Input: part model. Units: mm. Frame: model coordinates. Face numbers are marked on the shaded views. A direction names the side the tool comes from. Give positions to 0.01 mm unless a question says otherwise; leave off trailing zeros. Loops run counter-clockwise (first coordinate to the right, second up) from the corner with the lowest first, then second, coordinate; pieces in that order, holes last. Notation, with made-up numbers: (63, -6.5) -> (99, -6.5) arc R16 cw to (99, 13.5) -> close; hole circle Ø1 at (-28.75, -11). An arc over 180 degrees is marked (long way). Use CSV: the item, a comma, the result in double quotes.
```python
from build123d import *

# Parameters (mm, degrees)
SKETCH_1_R          = 10
SKETCH_1_R_2        = 1.5
EXTRUDE_1_DEPTH     = 4.2
SKETCH_2_R          = 10
SKETCH_2_R_2        = 4.5
SKETCH_2_R_3        = 1.5
SKETCH_2_R_4        = 2.5
CUT_EXTRUDE_1_DEPTH = 2.2


with BuildPart() as part:
    # 草图1 → 凸台-拉伸1 (new body)
    with BuildSketch(Plane(origin=(0, 0, 0), x_dir=(1, 0, 0), z_dir=(0, 1, 0))):
        Circle(SKETCH_1_R)
        with Locations((0, 6.5)):
            Circle(SKETCH_1_R_2, mode=Mode.SUBTRACT)
        with Locations((0, -6.5)):
            Circle(SKETCH_1_R_2, mode=Mode.SUBTRACT)
        with Locations((6.5, 0)):
            Circle(SKETCH_1_R_2, mode=Mode.SUBTRACT)
        with Locations((-6.5, 0)):
            Circle(SKETCH_1_R_2, mode=Mode.SUBTRACT)
        Circle(SKETCH_1_R_2, mode=Mode.SUBTRACT)
    extrude(amount=EXTRUDE_1_DEPTH)

    # 草图2 → 切除-拉伸1 (cut)
    with BuildSketch(Plane(origin=(0, 4.2, 0), x_dir=(1, 0, 0), z_dir=(0, 1, 0))):
        Circle(SKETCH_2_R)
        Circle(SKETCH_2_R_2, mode=Mode.SUBTRACT)
        with Locations((0, 6.5)):
            Circle(SKETCH_2_R_3, mode=Mode.SUBTRACT)
        with Locations((-6.5, 0)):
            Circle(SKETCH_2_R_3, mode=Mode.SUBTRACT)
        with Locations((0, -6.5)):
            Circle(SKETCH_2_R_3, mode=Mode.SUBTRACT)
        with Locations((6.5, 0)):
            Circle(SKETCH_2_R_3, mode=Mode.SUBTRACT)
        Circle(SKETCH_2_R_4)
        Circle(SKETCH_2_R_3, mode=Mode.SUBTRACT)
    extrude(amount=-CUT_EXTRUDE_1_DEPTH, mode=Mode.SUBTRACT)


solid = part.part
```
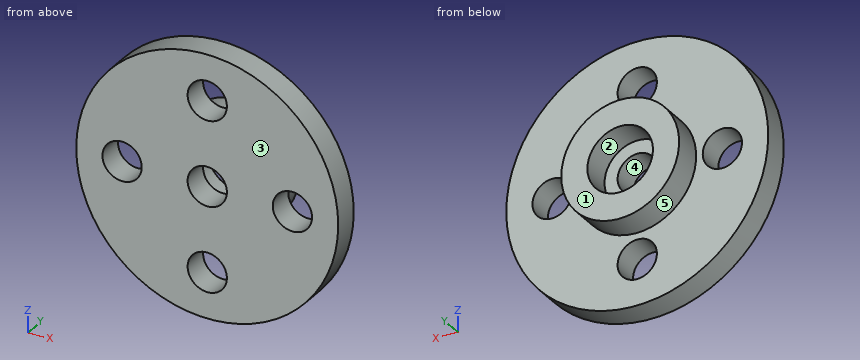
1) Ray query, line 1 (Z direction, x = 0, y = 1.5); line 2 (Z direction, x = -0.75, y = 1.3). Return the intervals inside material, ascending.
From the geometry:
line 1,"z = -10 to -8, -5 to -1.5, 1.5 to 5, 8 to 10"
line 2,"z = -9.97 to -7.8, -5.2 to -1.3, 1.3 to 5.2, 7.8 to 9.97"
2) Section query C-C (x = 6.5). Return loops of the section in (y, z).
From the geometry:
outline,"(0, -7.6) -> (2, -7.6) -> (2, -1.5) -> (0, -1.5) -> close; (0, 1.5) -> (2, 1.5) -> (2, 7.6) -> (0, 7.6) -> close"
3) Section query D-D (y = 3.65). Return loops of the section in (x, z), then the cut area to 3 significant figures.
From the geometry:
outline,"circle Ø9 at (0, 0); hole circle Ø5 at (0, 0)"
area,"44.0 mm^2"
4) Mould query, pull axis Z, two halves, no side actions, for the marked faces 3, 4 and 5. Classes: pulls with the +Z half, pulls with the -Z half, needs draft (parallel to the pull), parting line crosses it, or undercut.
From the geometry:
face 3,"needs draft"
face 4,"undercut"
face 5,"parting line crosses it"
5) Contact query for flat-ended pins moving along their axis: pin 1 (1.5 mm diameter, centred on x = -1, z = 0, fed in from +Y); pin 2 (1.5 mm diameter, centred on x = 1, z = 7.5, fed in from -Y); pin 3 (1 mm diameter, centred on y = 1, z = -7.5, fed in from +X); pin 4 (2 mm diameter, centred on y = 1, z = -4.5, fed in from -X). Output: stop coordinate, or through.
From the geometry:
pin 1,"stops at y = 2"
pin 2,"stops at y = 0"
pin 3,"stops at x = 7.14"
pin 4,"stops at x = -9.37"
6) Section query A-A (x = 0). Return loops of the section in (y, z).
From the geometry:
outline,"(0, -10) -> (2, -10) -> (2, -8) -> (0, -8) -> close; (0, -5) -> (2, -5) -> (2, -4.5) -> (4.2, -4.5) -> (4.2, -2.5) -> (2, -2.5) -> (2, -1.5) -> (0, -1.5) -> close; (0, 1.5) -> (2, 1.5) -> (2, 2.5) -> (4.2, 2.5) -> (4.2, 4.5) -> (2, 4.5) -> (2, 5) -> (0, 5) -> close; (0, 8) -> (2, 8) -> (2, 10) -> (0, 10) -> close"
7) Section query B-B (z = 0). Return loops of the section in (x, y).
From the geometry:
outline,"(-10, 0) -> (-8, 0) -> (-8, 2) -> (-10, 2) -> close; (-5, 0) -> (-1.5, 0) -> (-1.5, 2) -> (-2.5, 2) -> (-2.5, 4.2) -> (-4.5, 4.2) -> (-4.5, 2) -> (-5, 2) -> close; (1.5, 0) -> (5, 0) -> (5, 2) -> (4.5, 2) -> (4.5, 4.2) -> (2.5, 4.2) -> (2.5, 2) -> (1.5, 2) -> close; (8, 0) -> (10, 0) -> (10, 2) -> (8, 2) -> close"
8) Reachability of the marked faces 1 and 2 from +Z, -Z, +X, -X, +Y, -Y: full face, straight path, thin tool, end or side. Return the list, or none.
From the geometry:
face 1,"+Z, -Z, +X, -X, +Y"
face 2,"+Y"
